```python
from build123d import *

# Parameters (mm, degrees)
SKETCH1_W               = 38.1
SKETCH1_H               = 69.85
SKETCH1_R               = 3.302
SKETCH1_R_2             = 1.651
BOSS_EXTRUDE1_DEPTH     = 6.35
SKETCH2_W               = 19.05
SKETCH2_H               = 11.43
CUT_EXTRUDE1_DEPTH      = 2.54
CUT_EXTRUDE2_DEPTH      = 70.390828962
CUT_EXTRUDE2_DEPTH_BACK = 70.390828962
SKETCH5_W               = 2.54
SKETCH5_H               = 1.27
SKETCH6_W               = 2.54
SKETCH6_H               = 15.24
CUT_EXTRUDE3_DEPTH      = 1.016
SKETCH7_W               = 38.1
SKETCH7_H               = 18.542
CUT_EXTRUDE4_DEPTH      = 1.524


with BuildPart() as part:
    # Sketch1 → Boss-Extrude1 (new body)
    with BuildSketch(Plane(origin=(0, 0, 0), x_dir=(1, 0, 0), z_dir=(0, 1, 0))):
        with Locations((6.35, 29.337)):
            Rectangle(SKETCH1_W, SKETCH1_H)
        with Locations(Location((0, 0, 0), (0, 0, 270))):
            Circle(SKETCH1_R, mode=Mode.SUBTRACT)
        with Locations(Location((0, 58.674, 0), (0, 0, 270))):
            Circle(SKETCH1_R, mode=Mode.SUBTRACT)
        with Locations(Location((18.161, 59.309, 0), (0, 0, 270))):
            Circle(SKETCH1_R_2, mode=Mode.SUBTRACT)
        with Locations(Location((18.161, -1.143, 0), (0, 0, 270))):
            Circle(SKETCH1_R_2, mode=Mode.SUBTRACT)
    extrude(amount=BOSS_EXTRUDE1_DEPTH)

    # Sketch2 → Cut-Extrude1 (cut)
    with BuildSketch(Plane(origin=(0, 6.35, 0), x_dir=(1, 0, 0), z_dir=(0, 1, 0))):
        with Locations((9.525, 12.827)):
            Rectangle(SKETCH2_W, SKETCH2_H)
    extrude(amount=-CUT_EXTRUDE1_DEPTH, mode=Mode.SUBTRACT)

    # Sketch5 → Cut-Extrude2 (cut, two sides: drawn at the far end of the back side and taken through both)
    with BuildSketch(Plane(origin=(0, 6.35, 0), x_dir=(1, 0, 0), z_dir=(0, 1, 0)).offset(-CUT_EXTRUDE2_DEPTH_BACK)):
        with Locations((10.16, 21.082)):
            Rectangle(SKETCH5_W, SKETCH5_H)
        with Locations((10.16, 4.572)):
            Rectangle(SKETCH5_W, SKETCH5_H)
    extrude(amount=CUT_EXTRUDE2_DEPTH + CUT_EXTRUDE2_DEPTH_BACK, mode=Mode.SUBTRACT)

    # Sketch6 → Cut-Extrude3 (cut)
    with BuildSketch(Plane.XZ):
        with Locations((10.16, -12.827)):
            Rectangle(SKETCH6_W, SKETCH6_H)
    extrude(amount=-CUT_EXTRUDE3_DEPTH, mode=Mode.SUBTRACT)

    # Sketch7 → Cut-Extrude4 (cut)
    with BuildSketch(Plane(origin=(0, 6.35, 0), x_dir=(1, 0, 0), z_dir=(0, 1, 0))):
        with Locations((6.35, 43.561)):
            Rectangle(SKETCH7_W, SKETCH7_H)
    extrude(amount=-CUT_EXTRUDE4_DEPTH, mode=Mode.SUBTRACT)


solid = part.part
```
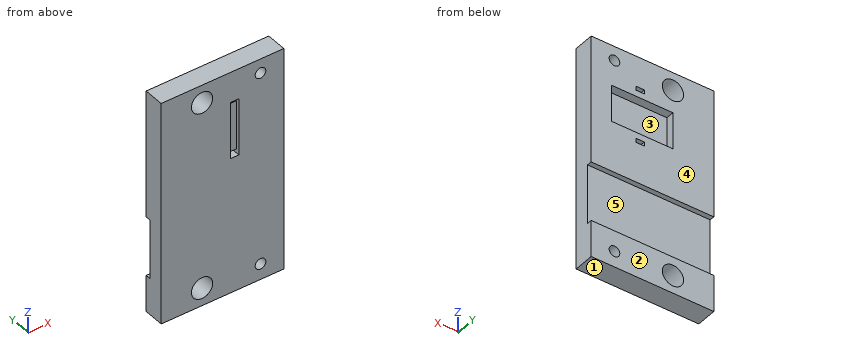
Here's how the part is built. I have some questions about the finished solid (model axes, mm). Face numbers are marked on the shaded views. A direction names the side the tool comes from. Coordinates: 2 decimals unless noted, no trailing zeros. Order: outer loops, then holes, each group sorted by start corner. A loop starts at its lowest first (then second) coordinate and runs counter-clockwise, first axis right, second up.
1) Imagine slicing it at C-C on x = -7. List the corners of the cut face in (y, z) for me.
2) Imagine slicing it at A-A on x = 5.5. List the corners of the cut face in (y, z) for me.
3) Imagine slicing it at D-D on z = -40.5. List the corners of the cut face in (x, y) for me.
4) Will these pins go through, and if not, where does the flat tip stop? pin 1 (1.3 mm diameter, centred on x = 10.5, z = -12, fed in from -Y); pin 2 (3 mm diameter, centred on x = -3, z = -38, fed in from +Y).
5) Which directions (+Z, -Z, +X, -X, +Y, -Y) give clear straight access to the entire face, cutting with the end or side of a thin tool? Please do the marked faces 4 and 5.
6) Imagine slicing it at B-B on y = 2.5. List the corners of the cut face in (x, z) for me.
7) We'd pull the mould along Z, two halves only. Please class the marked faces 1, 2 and 3: +Z half, -Z half, draft (parallel to the pull), parting line (faces both ways), or undercut.
8) I need wall thicknesses on line 1 (Z direction, x = -4, y = 5); line 2 (X direction, y = 4.5, z = 0); line 3 (X direction, y = 5.75, z = -13). Which ranges of each line are inside material? Lowest first, please.
Response values:
1. outline: (0, -64.26) - (6.35, -64.26) - (6.35, -52.83) - (4.83, -52.83) - (4.83, -34.29) - (6.35, -34.29) - (6.35, 5.59) - (0, 5.59) - close
2. outline: (0, -64.26) - (6.35, -64.26) - (6.35, -52.83) - (4.83, -52.83) - (4.83, -34.29) - (6.35, -34.29) - (6.35, -18.54) - (3.81, -18.54) - (3.81, -7.11) - (6.35, -7.11) - (6.35, 5.59) - (0, 5.59) - close
3. outline: (-12.7, 0) - (25.4, 0) - (25.4, 4.83) - (-12.7, 4.83) - close
4. pin 1: stops at y = 1.02
4. pin 2: stops at y = 4.83
5. face 4: +Z, -Z, +X, -X, +Y
5. face 5: +X, -X, +Y
6. outline: (-12.7, -64.26) - (25.4, -64.26) - (25.4, 5.59) - (-12.7, 5.59) - close; hole circle Ø6.6 at (0, -58.67); hole circle Ø6.6 at (0, 0); hole (8.89, -21.72) - (11.43, -21.72) - (11.43, -20.45) - (8.89, -20.45) - close; hole (8.89, -5.21) - (11.43, -5.21) - (11.43, -3.94) - (8.89, -3.94) - close; hole circle Ø3.3 at (18.16, -59.31); hole circle Ø3.3 at (18.16, 1.14)
7. face 1: -Z half
7. face 2: draft
7. face 3: undercut
8. line 1: z = -64.26 to -52.83, -34.29 to 5.59
8. line 2: x = -12.7 to -3.3, 3.3 to 16.97, 19.35 to 25.4
8. line 3: x = -12.7 to 0, 19.05 to 25.4
